Design review of the part built by this model. Coordinates are the model's own, in mm. A direction names the side the tool comes from. Coordinates: 2 decimals unless noted, no trailing zeros. Write each loop counter-clockwise with the first axis right and the second up, starting at its lowest first coordinate (ties: lowest second). Pieces come first, ordered by that corner, then holes.
Q1. For faces 5 (the flat face through (-426, 9.525, 26)), 6 (the flat face through (-435, 0, -95.25)), list the 3-axis set-ups (+Z, -Z, +X, -X, +Y, -Y) from which the entire face can be reached by the end or side of a thin tool; tool diameter is ignored.
Q2. Take a section at A-A, the plane z = -48.5. Write out the cut boundary in (x, y) (3 decimals).
Q3. Take a section at C-C, the plane x = -247. Write out the cut boundary in (y, z) (3 decimals).
Q4. For L1, parallel to Z at x = -551.5, y = -7.5; L2, parallel to X at y = 3.75, z = -28.5, list the stretches that pass through material, from the lowest coordinate up.
Q5. The part is to be moulded in two halves that separate along Z. For faces 1 (the flat face through (-426, 0, -127)), 2 (the flat face through (-426, 0, 127)), 3 (the flat face through (-426, -9.525, 26)), 4 (the flat face through (-203.2, 0, -36)), say which applies: released by +Z, released by -Z, zero draft, split by the parting line, or undercut.
Q6. Take a section at B-B, the plane y = 6.5. Write out the cut boundary in (x, z).
from build123d import *

# Parameters (mm, degrees)
F0_W     = 19.05
F0_H     = 254
F1_DEPTH = 863.6
F2_W     = 457.2
F2_H     = 120.65
F3_DEPTH = 19.051


with BuildPart() as f1:
    # F0 (on Right) → F1 (new body)
    with BuildSketch(Plane.YZ):
        Rectangle(F0_W, F0_H)
    extrude(amount=-F1_DEPTH)

    # F2 (on face) → F3 (cut, through all)
    with BuildSketch(Plane.XZ.offset(9.525)):
        with Locations((-431.8, -34.925)):
            Rectangle(F2_W, F2_H)
    extrude(amount=-F3_DEPTH, mode=Mode.SUBTRACT)


solid = f1.part
Responses:
1. face 5: +Z, -Z, +X, -X, +Y
1. face 6: +Y, -Y
2. outline: (-863.6, -9.525) - (-660.4, -9.525) - (-660.4, 9.525) - (-863.6, 9.525) - close; (-203.2, -9.525) - (0, -9.525) - (0, 9.525) - (-203.2, 9.525) - close
3. outline: (-9.525, -127) - (9.525, -127) - (9.525, -95.25) - (-9.525, -95.25) - close; (-9.525, 25.4) - (9.525, 25.4) - (9.525, 127) - (-9.525, 127) - close
4. L1: z = -127 to -95.25, 25.4 to 127
4. L2: x = -863.6 to -660.4, -203.2 to 0
5. face 1: released by -Z
5. face 2: released by +Z
5. face 3: zero draft
5. face 4: undercut
6. outline: (-863.6, -127) - (0, -127) - (0, 127) - (-863.6, 127) - close; hole (-660.4, -95.25) - (-203.2, -95.25) - (-203.2, 25.4) - (-660.4, 25.4) - close
